Design review of the part built by this model. Coordinates are the model's own, in mm. A direction names the side the tool comes from. Give positions to 0.01 mm unless a question says otherwise; leave off trailing zeros. Write each loop counter-clockwise with the first axis right and the second up, starting at its lowest first coordinate (ties: lowest second). Pieces come first, ordered by that corner, then holes. Notation, with made-up numbers: (8.5, 86.25) -> (47.5, 86.25) arc R17 ccw to (47.5, 112.25) -> close; hole circle Ø2 at (11.25, 85). An arc over 180 degrees is marked (long way). Use CSV: the item, a comma, the result in double quotes.
```python
from build123d import *

# Parameters (mm, degrees)
SKETCH1_W            = 64.135
SKETCH1_H            = 127
BOSS_EXTRUDE1_DEPTH  = 6.35
BOSS_EXTRUDE13_DEPTH = 8.89
BOSS_EXTRUDE14_DEPTH = 8.5725
BOSS_EXTRUDE15_DEPTH = 6.985
BOSS_EXTRUDE16_DEPTH = 5.3975
BOSS_EXTRUDE17_START = 12.3825
BOSS_EXTRUDE17_DEPTH = 6.985
BOSS_EXTRUDE18_START = 27.94
BOSS_EXTRUDE18_DEPTH = 13.335
BOSS_EXTRUDE19_DEPTH = 27.94
BOSS_EXTRUDE20_START = 69.215
BOSS_EXTRUDE20_DEPTH = 13.97
BOSS_EXTRUDE21_START = 41.91
BOSS_EXTRUDE21_DEPTH = 28.575
BOSS_EXTRUDE22_START = 111.76
BOSS_EXTRUDE22_DEPTH = 6.35
SKETCH18_R           = 2.54
SKETCH18_W           = 19.3675
SKETCH18_H           = 127
CUT_EXTRUDE5_DEPTH   = 7.35
SKETCH20_W           = 1.905
SKETCH20_H           = 5.08
FILLET3_R            = 2.54


with BuildPart() as part:
    # Sketch1 → Boss-Extrude1 (new body)
    with BuildSketch(Plane(origin=(0, 0, 0), x_dir=(1, 0, 0), z_dir=(0, 1, 0))):
        Rectangle(SKETCH1_W, SKETCH1_H)
    extrude(amount=BOSS_EXTRUDE1_DEPTH)

    # Sketch12 → Boss-Extrude13 (add)
    with BuildSketch(Plane(origin=(0, 0, -63.5), x_dir=(-1, 0, 0), z_dir=(0, 0, -1))):
        Polygon((-37.660740352, -11.181831339), (-37.09962, -4.768196367), (-26.965439184, -0.042550244), (-17.805819185, -6.456185215), (-18.219259648, -11.181831339), (-11.455819185, -11.181831339), (-11.455819185, 6.35), (-28.281950999, 6.35), (-43.105928196, -0.562534091), (-44.03499632, -11.181831339), align=None)
    extrude(amount=-BOSS_EXTRUDE13_DEPTH)

    # Sketch13 → Boss-Extrude14 (add)
    with BuildSketch(Plane.XY.offset(-54.61)):
        with BuildLine():
            Line((44.03499632, -11.181831339), (34.29, -11.181831339))
            ThreePointArc((34.29, -11.181831339), (27.94, -4.831831339), (21.59, -11.181831339))
            Line((21.59, -11.181831339), (11.455819185, -11.181831339))
            Line((11.455819185, -11.181831339), (11.455819185, 0))
            Line((11.455819185, 0), (32.0675, 0))
            Line((32.0675, 0), (32.0675, 4.584769511))
            Line((32.0675, 4.584769511), (43.105928196, -0.562534091))
            Line((43.105928196, -0.562534091), (44.03499632, -11.181831339))
        make_face()
    extrude(amount=BOSS_EXTRUDE14_DEPTH)

    # Sketch14 → Boss-Extrude15 (add)
    with BuildSketch(Plane.XY.offset(-46.0375)):
        with BuildLine():
            Line((34.925, -11.181831339), (44.03499632, -11.181831339))
            Line((44.03499632, -11.181831339), (43.105928196, -0.562534091))
            Line((43.105928196, -0.562534091), (32.0675, 4.584769511))
            Line((32.0675, 4.584769511), (32.0675, 0))
            Line((32.0675, 0), (11.455819185, 0))
            Line((11.455819185, 0), (11.455819185, -11.181831339))
            Line((11.455819185, -11.181831339), (20.955, -11.181831339))
            ThreePointArc((20.955, -11.181831339), (27.94, -4.196831339), (34.925, -11.181831339))
        make_face()
    extrude(amount=BOSS_EXTRUDE15_DEPTH)

    # Sketch15 → Boss-Extrude16 (add)
    with BuildSketch(Plane.XY.offset(-39.0525)):
        with BuildLine():
            Line((36.03625, -11.181831339), (44.03499632, -11.181831339))
            Line((44.03499632, -11.181831339), (43.105928196, -0.562534091))
            Line((43.105928196, -0.562534091), (32.0675, 4.584769511))
            Line((32.0675, 4.584769511), (32.0675, 0))
            Line((32.0675, 0), (11.455819185, 0))
            Line((11.455819185, 0), (11.455819185, -11.181831339))
            Line((11.455819185, -11.181831339), (19.84375, -11.181831339))
            ThreePointArc((19.84375, -11.181831339), (27.94, -3.085581339), (36.03625, -11.181831339))
        make_face()
    extrude(amount=BOSS_EXTRUDE16_DEPTH)

    # Sketch14_2 → Boss-Extrude17 (add)
    with BuildSketch(Plane.XY.offset(-46.0375).offset(BOSS_EXTRUDE17_START)):
        with BuildLine():
            Line((34.925, -11.181831339), (44.03499632, -11.181831339))
            Line((44.03499632, -11.181831339), (43.105928196, -0.562534091))
            Line((43.105928196, -0.562534091), (32.0675, 4.584769511))
            Line((32.0675, 4.584769511), (32.0675, 0))
            Line((32.0675, 0), (11.455819185, 0))
            Line((11.455819185, 0), (11.455819185, -11.181831339))
            Line((11.455819185, -11.181831339), (20.955, -11.181831339))
            ThreePointArc((20.955, -11.181831339), (27.94, -4.196831339), (34.925, -11.181831339))
        make_face()
    extrude(amount=BOSS_EXTRUDE17_DEPTH)

    # Sketch13_2 → Boss-Extrude18 (add)
    with BuildSketch(Plane.XY.offset(-54.61).offset(BOSS_EXTRUDE18_START)):
        with BuildLine():
            Line((44.03499632, -11.181831339), (34.29, -11.181831339))
            ThreePointArc((34.29, -11.181831339), (27.94, -4.831831339), (21.59, -11.181831339))
            Line((21.59, -11.181831339), (11.455819185, -11.181831339))
            Line((11.455819185, -11.181831339), (11.455819185, 0))
            Line((11.455819185, 0), (32.0675, 0))
            Line((32.0675, 0), (32.0675, 4.584769511))
            Line((32.0675, 4.584769511), (43.105928196, -0.562534091))
            Line((43.105928196, -0.562534091), (44.03499632, -11.181831339))
        make_face()
    extrude(amount=BOSS_EXTRUDE18_DEPTH)

    # Sketch16 → Boss-Extrude19 (add)
    with BuildSketch(Plane.XY.offset(-13.335)):
        Polygon((20.6375, -11.181831339), (20.6375, -3.879331339), (35.2425, -3.879331339), (35.2425, -11.181831339), (44.03499632, -11.181831339), (43.105928196, -0.562534091), (32.0675, 4.584769511), (32.0675, 0), (11.455819185, 0), (11.455819185, -11.181831339), align=None)
    extrude(amount=BOSS_EXTRUDE19_DEPTH)

    # Sketch13_3 → Boss-Extrude20 (add)
    with BuildSketch(Plane.XY.offset(-54.61).offset(BOSS_EXTRUDE20_START)):
        with BuildLine():
            Line((44.03499632, -11.181831339), (34.29, -11.181831339))
            ThreePointArc((34.29, -11.181831339), (27.94, -4.831831339), (21.59, -11.181831339))
            Line((21.59, -11.181831339), (11.455819185, -11.181831339))
            Line((11.455819185, -11.181831339), (11.455819185, 0))
            Line((11.455819185, 0), (32.0675, 0))
            Line((32.0675, 0), (32.0675, 4.584769511))
            Line((32.0675, 4.584769511), (43.105928196, -0.562534091))
            Line((43.105928196, -0.562534091), (44.03499632, -11.181831339))
        make_face()
    extrude(amount=BOSS_EXTRUDE20_DEPTH)

    # Sketch16_2 → Boss-Extrude21 (add)
    with BuildSketch(Plane.XY.offset(-13.335).offset(BOSS_EXTRUDE21_START)):
        Polygon((20.6375, -11.181831339), (20.6375, -3.879331339), (35.2425, -3.879331339), (35.2425, -11.181831339), (44.03499632, -11.181831339), (43.105928196, -0.562534091), (32.0675, 4.584769511), (32.0675, 0), (11.455819185, 0), (11.455819185, -11.181831339), align=None)
    extrude(amount=BOSS_EXTRUDE21_DEPTH)

    # Sketch13_4 → Boss-Extrude22 (add)
    with BuildSketch(Plane.XY.offset(-54.61).offset(BOSS_EXTRUDE22_START)):
        with BuildLine():
            Line((44.03499632, -11.181831339), (34.29, -11.181831339))
            ThreePointArc((34.29, -11.181831339), (27.94, -4.831831339), (21.59, -11.181831339))
            Line((21.59, -11.181831339), (11.455819185, -11.181831339))
            Line((11.455819185, -11.181831339), (11.455819185, 0))
            Line((11.455819185, 0), (32.0675, 0))
            Line((32.0675, 0), (32.0675, 4.584769511))
            Line((32.0675, 4.584769511), (43.105928196, -0.562534091))
            Line((43.105928196, -0.562534091), (44.03499632, -11.181831339))
        make_face()
    extrude(amount=BOSS_EXTRUDE22_DEPTH)

    # Sketch18 → Cut-Extrude5 (cut, through all)
    with BuildSketch(Plane.XZ):
        with Locations((0, 12.7)):
            Circle(SKETCH18_R)
        with Locations((0, -38.1)):
            Circle(SKETCH18_R)
        with Locations((-22.38375, 0)):
            Rectangle(SKETCH18_W, SKETCH18_H)
    extrude(amount=-CUT_EXTRUDE5_DEPTH, mode=Mode.SUBTRACT)

    # Sketch20 → Cut-Revolve1 (revolve, cut)
    with BuildSketch(Plane.XZ.offset(11.181831339)):
        with Locations((16.522909592, -50.32375)):
            Rectangle(SKETCH20_W, SKETCH20_H)
        with Locations((16.522909592, 26.035)):
            Rectangle(SKETCH20_W, SKETCH20_H)
    revolve(axis=Axis((27.94, -11.181831339, 63.5), (0, 0, -1)), mode=Mode.SUBTRACT)

    # Fillet3
    fillet3_edges = [part.edges().sort_by_distance(p)[0] for p in [
        (11.455819185, 0, 0),
        (43.105928196, -0.562534091, 0),
        (44.03499632, -11.181831339, 0),
        (32.0675, 4.584769511, 0),
        (11.455819185, -11.181831339, 0),
        (-12.7, 0, 0),
    ]]
    fillet(fillet3_edges, radius=FILLET3_R)


solid = part.part
```
(1) For line 1 along Z through (x, y) = (0, 4.75); line 2 along Z through (x, y) = (34.5, -1) (3 decimals); line 3 along X through (y, z) = (-8.5, 55.5), list the stretches that pass through material, from the lowest coordinate up. Write a range as [from, to].
Established:
line 1,"z = [-63.5, -40.64], [-35.56, 10.16], [15.24, 63.5]"
line 2,"z = [-63.5, -52.864], [-47.784, 23.495], [28.575, 63.5]"
line 3,"x = [11.46, 20.64], [35.24, 43.8]"
(2) Take a section at C-C (z = 51). Write out the cut boundary in (x, y).
Established:
outline,"(-12.7, 2.54) arc R2.54 ccw to (-10.16, 0) -> (8.92, 0) arc R2.54 cw to (11.46, -2.54) -> (11.46, -8.64) arc R2.54 ccw to (14, -11.18) -> (20.64, -11.18) -> (20.64, -3.88) -> (35.24, -3.88) -> (35.24, -11.18) -> (41.26, -11.18) arc R2.54 ccw to (43.79, -8.42) -> (43.23, -2.02) arc R2.54 ccw to (41.78, 0.06) -> (33.53, 3.9) arc R2.54 cw to (32.07, 6.2) -> (32.07, 6.35) -> (-12.7, 6.35) -> close"
(3) Clearance check with flat-ended pins moving along their axes: pin 1 (5 mm diameter, centred on y = -6, z = 22.5, fed in from +X); pin 2 (2 mm diameter, centred on y = 0.5, z = 27, fed in from +X); pin 3 (7.5 mm diameter, centred on x = 28, z = 47.5, fed in from -Y). State where each tip first meets the part, or that it passes through.
Established:
pin 1,"stops at x = 43.8"
pin 2,"stops at x = 42.55"
pin 3,"stops at y = -3.88"
(4) Tool access review of faces 5 (the face through (18.01, -8.79, -59.12)), 6 (the face through (11.456, -6, -1)), 7 (the face through (16, 0, -63.5)), 8 (the face through (28.08, -4.833, -50.384)), 9 (the face through (29, -4, -39.052)): name each direction out of +Z, -Z, +X, -X, +Y, -Y from which nothing blocks a thin tool from reaching the whole face with its end or side.
Established:
face 5,"-Z"
face 6,"+Z, -Z, -X, -Y"
face 7,"-Z, +X, -X, +Y, -Y"
face 8,"+Z, -Z, -Y"
face 9,"-Y"
(5) Mouldability with a two-part tool opening along X and no side actions: class faces 1 (the face through (27, 0, 23.495)), 2 (the face through (-11.976, 0.764, 0.889)), 3 (the face through (28, -4.6, -46.038)), 4 (the face through (38, -11.182, -1)) as +X half, -X half, draft (parallel to the pull), parting line (faces both ways), or undercut.
Established:
face 1,"undercut"
face 2,"-X half"
face 3,"undercut"
face 4,"draft"
(6) Take a section at B-B (x = 0). Write out the cut boundary in (y, z), then the cut area to 3 significant figures.
Established:
outline,"(0, -63.5) -> (6.35, -63.5) -> (6.35, -40.64) -> (0, -40.64) -> close; (0, -35.56) -> (6.35, -35.56) -> (6.35, 10.16) -> (0, 10.16) -> close; (0, 15.24) -> (6.35, 15.24) -> (6.35, 63.5) -> (0, 63.5) -> close"
area,"742 mm2"
(7) Take a section at A-A (z = 12.7). Write out the cut boundary in (x, y).
Established:
outline,"(-12.7, 2.54) arc R2.54 ccw to (-10.16, 0) -> (-2.54, 0) -> (-2.54, 6.35) -> (-12.7, 6.35) -> close; (2.54, 0) -> (8.92, 0) arc R2.54 cw to (11.46, -2.54) -> (11.46, -8.64) arc R2.54 ccw to (14, -11.18) -> (20.64, -11.18) -> (20.64, -3.88) -> (35.24, -3.88) -> (35.24, -11.18) -> (41.26, -11.18) arc R2.54 ccw to (43.79, -8.42) -> (43.23, -2.02) arc R2.54 ccw to (41.78, 0.06) -> (33.53, 3.9) arc R2.54 cw to (32.07, 6.2) -> (32.07, 6.35) -> (2.54, 6.35) -> close"
